```python
from build123d import *

# Parameters (mm, degrees)
BOSS_EXTRUDE1_DEPTH = 36
SKETCH2_OUTSIDE_W   = 53.43
SKETCH2_OUTSIDE_H   = 77.43
SKETCH2_OUTSIDE_R   = 1
CUT_EXTRUDE2_DEPTH  = 5
SKETCH3_R           = 7.5
CUT_EXTRUDE3_DEPTH  = 5
SKETCH4_R           = 4
SKETCH4_R_2         = 1
CUT_EXTRUDE5_DEPTH  = 5


with BuildPart() as part:
    # Sketch1 → Boss-Extrude1 (new body)
    with BuildSketch(Plane.XY):
        Polygon((0, 0), (-10.5, 0), (-10.5, -35), (18, -35), (18, 23), (20, 23), (20, -37), (-12.5, -37), (-12.5, 2), (0, 2), align=None)
    extrude(amount=BOSS_EXTRUDE1_DEPTH)

    # Sketch2 outside → Cut-Extrude2 (cut)
    # profile 1 of 4: a face of its own
    with BuildSketch(Plane(origin=(20, 0, 0), x_dir=(0, 0, -1), z_dir=(1, 0, 0))):
        with Locations((-18, -7)):
            Rectangle(SKETCH2_OUTSIDE_W, SKETCH2_OUTSIDE_H)
        with BuildLine():
            Line((-27.403498968, 23), (-8.191734442, 23))
            ThreePointArc((-8.191734442, 23), (-6.991166755, 22.599574078), (-6.271337492, 21.55863723))
            Line((-6.271337492, 21.55863723), (-0.398015251, 1.368235471))
            ThreePointArc((-0.398015251, 1.368235471), (-0.100003851, -0.014250056), (0, -1.424950681))
            Line((0, -1.424950681), (0, -37))
            Line((0, -37), (-36, -37))
            Line((-36, -37), (-36, -1.512851617))
            ThreePointArc((-36, -1.512851617), (-35.887491609, -0.01702085), (-35.552498063, 1.445151214))
            Line((-35.552498063, 1.445151214), (-29.313998581, 21.591600566))
            ThreePointArc((-29.313998581, 21.591600566), (-28.590259025, 22.609844889), (-27.403498968, 23))
        make_face(mode=Mode.SUBTRACT)
    # profile 2 of 4: a face of its own
    with BuildSketch(Plane(origin=(20, 0, 0), x_dir=(0, 0, -1), z_dir=(1, 0, 0))):
        with Locations((-17.797616705, 6.5)):
            Circle(SKETCH2_OUTSIDE_R)
    # profile 3 of 4: a face of its own
    with BuildSketch(Plane(origin=(20, 0, 0), x_dir=(0, 0, -1), z_dir=(1, 0, 0))):
        with Locations((-22.797616705, 13)):
            Circle(SKETCH2_OUTSIDE_R)
    # profile 4 of 4: a face of its own
    with BuildSketch(Plane(origin=(20, 0, 0), x_dir=(0, 0, -1), z_dir=(1, 0, 0))):
        with Locations((-12.797616705, 13)):
            Circle(SKETCH2_OUTSIDE_R)
    extrude(amount=-CUT_EXTRUDE2_DEPTH, mode=Mode.SUBTRACT)

    # Sketch3 → Cut-Extrude3 (cut)
    with BuildSketch(Plane.ZY.offset(12.5)):
        with Locations((18, -17.5)):
            Circle(SKETCH3_R)
    extrude(amount=-CUT_EXTRUDE3_DEPTH, mode=Mode.SUBTRACT)

    # Sketch4 → Cut-Extrude5 (cut)
    with BuildSketch(Plane.XZ.offset(37)):
        with Locations(Location((3.75, 18, 0), (0, 0, 270))):
            Circle(SKETCH4_R)
        with Locations(Location((3.75, 12, 0), (0, 0, 270))):
            Circle(SKETCH4_R_2)
        with Locations(Location((3.75, 24, 0), (0, 0, 270))):
            Circle(SKETCH4_R_2)
        with Locations(Location((9.75, 18, 0), (0, 0, 270))):
            Circle(SKETCH4_R_2)
        with Locations(Location((-2.25, 18, 0), (0, 0, 270))):
            Circle(SKETCH4_R_2)
    extrude(amount=-CUT_EXTRUDE5_DEPTH, mode=Mode.SUBTRACT)


solid = part.part
```
Geometry: final body of the model. Coordinates: model frame, mm. A direction names the side the tool comes from. Coordinates: 2 decimals unless noted, no trailing zeros. Order: outer loops, then holes, each group sorted by start corner. A loop starts at its lowest first (then second) coordinate and runs counter-clockwise, first axis right, second up. Notation, with made-up numbers: (-22.75, 28) - (3.25, 28) arc R9 cw to (3.25, 40) - close; hole circle Ø3 at (-22.5, 64). An arc over 180 degrees is marked (long way). Return JSON: item names as keys, results as strings. Group by question number.
1. Cut plane D-D (x = -8). Output: boundary loops of the cut face in (y, z), plus the area to 3 significant figures.
2. Pin query (flat end, axial travel): pin 1 (8 mm diameter, centred on x = -4.5, z = 26, fed in from +Y); pin 2 (1 mm diameter, centred on y = 7, z = 7, fed in from -X); pin 3 (8.5 mm diameter, centred on x = 6, z = 16.5, fed in from +Y); pin 4 (1.6 mm diameter, centred on y = 6.5, z = 17.8, fed in from -X). Return the tip coordinate at first contact, or that it passes through.
3. Cut plane B-B (x = -2.25). Output: boundary loops of the cut face in (y, z), plus the area to 3 significant figures.
4. Material intervals for line 1 along X through (y, z) = (-36.4, 18); line 2 along Y through (x, z) = (-10, 18); line 3 along X through (y, z) = (-32, 6.5), sorted ascending. Write a range as [from, to].
5. Pull-direction query (Y, two-part tool) for faces 1 (the face through (4.426, -36.014, 12.737)), 2 (the face through (19.014, 12.024, 13.014)), 3 (the face through (-6, 2, 18)); classes: pulls with the +Y half, pulls with the -Y half, needs draft (parallel to the pull), parting line crosses it, or undercut.
6. Cut plane A-A (y = -17.5). Output: boundary loops of the cut face in (x, z).
7. Cut plane C-C (x = 3.75). Output: boundary loops of the cut face in (y, z), plus the area to 3 significant figures.
8. Set-up query: faces 4 (the face through (-5, 0, 18)), 5 (the face through (-11.5, -12.4, 12.5)), 6 (the face through (18, -6, 18)). Return all of +Z, -Z, +X, -X, +Y, -Y with unobstructed straight access to the full face (end or side cutting, diameter ignored); none if empty.
Resolved:
{
 "1": {"outline": "(-37, 0) - (-35, 0) - (-35, 36) - (-37, 36) - close; (0, 0) - (2, 0) - (2, 36) - (0, 36) - close", "area": "144 mm²"},
 "2": {"pin 1": "stops at y = 2", "pin 2": "stops at x = 18", "pin 3": "stops at y = -35", "pin 4": "passes through"},
 "3": {"outline": "(-37, 0) - (-35, 0) - (-35, 17) - (-37, 17) - close; (-37, 19) - (-35, 19) - (-35, 36) - (-37, 36) - close; (0, 0) - (2, 0) - (2, 36) - (0, 36) - close", "area": "140 mm²"},
 "4": {"line 1": "x = [-12.5, -3.25], [-1.25, -0.25], [7.75, 8.75], [10.75, 20]", "line 2": "y = [-37, -35], [0, 2]", "line 3": "x = [-12.5, -10.5], [18, 20]"},
 "5": {"face 1": "needs draft", "face 2": "undercut", "face 3": "pulls with the +Y half"},
 "6": {"outline": "(-12.5, 0) - (-10.5, 0) - (-10.5, 10.5) - (-12.5, 10.5) - close; (-12.5, 25.5) - (-10.5, 25.5) - (-10.5, 36) - (-12.5, 36) - close; (18, 0) - (20, 0) - (20, 36) - (18, 36) - close"},
 "7": {"outline": "(-37, 0) - (-35, 0) - (-35, 11) - (-37, 11) - close; (-37, 13) - (-35, 13) - (-35, 14) - (-37, 14) - close; (-37, 22) - (-35, 22) - (-35, 23) - (-37, 23) - close; (-37, 25) - (-35, 25) - (-35, 36) - (-37, 36) - close", "area": "48.0 mm²"},
 "8": {"face 4": "+Z, -Z", "face 5": "-X", "face 6": "+Z, -Z, +Y"}
}
